Geometry check sheet. Reference: drawing and pictorial views, mm from the part's lowest x, y, z. A direction names the side the tool comes from. Give positions to 0.01 mm unless a question says otherwise; leave off trailing zeros. Write each loop counter-clockwise with the first axis right and the second up, starting at its lowest first coordinate (ties: lowest second). Pieces come first, ordered by that corner, then holes. Notation, with made-up numbers: (-11.5, 86.5) -> (17.5, 86.5) arc R29 cw to (17.5, 106.5) -> close; hole circle Ø2 at (77.5, -5.75). An arc over 180 degrees is marked (long way). Return JSON: item names as keys, results as strings.
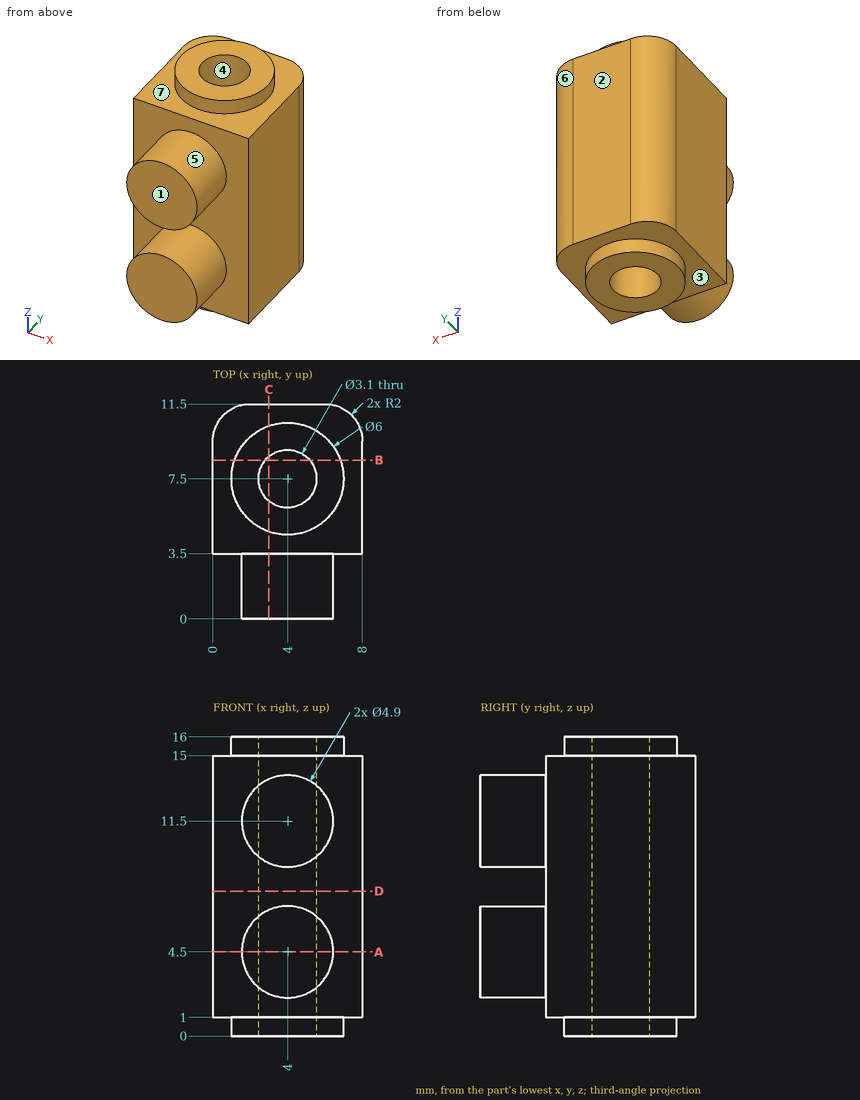
(1) Cross-section at D-D on z = 7.75. Enter the section's corners in (x, y).
Reply:
{"outline": "(0, 3.5) -> (8, 3.5) -> (8, 9.5) arc R2 ccw to (6, 11.5) -> (2, 11.5) arc R2 ccw to (0, 9.5) -> close; hole circle Ø3.1 at (4, 7.5)"}
(2) Cross-section at B-B on y = 8.5. Enter the section's corners in (x, z), then the cut area to 3 significant figures.
Reply:
{"outline": "(0, 1) -> (1.17, 1) -> (1.17, 0) -> (2.82, 0) -> (2.82, 16) -> (1.17, 16) -> (1.17, 15) -> (0, 15) -> close; (5.18, 0) -> (6.83, 0) -> (6.83, 1) -> (8, 1) -> (8, 15) -> (6.83, 15) -> (6.83, 16) -> (5.18, 16) -> close", "area": "85.4 mm^2"}
(3) Thickness scan on L1, parallel to Y at x = 4, z = 12; L2, parallel to Y at x = 2.75, z = 9; L3, parallel to X at y = 6.75, z = 13. Record the ranges inside material, lowest first.
Reply:
{"L1": "0 to 5.95, 9.05 to 11.5", "L2": "3.5 to 6.58, 8.42 to 11.5", "L3": "0 to 2.64, 5.36 to 8"}
(4) Set-up check for the marked faces 5, 6 and 7: record each of +Z, -Z, +X, -X, +Y, -Y from which the full face is reachable in a straight line by a thin tool's end or side.
Reply:
{"face 5": "-Y", "face 6": "+Z, -Z, +X, +Y", "face 7": "+Z"}
(5) Release check for a two-part mould opening along Y. For the marked faces 1, 2, 3 and 4 record: pulls with the +Y half, pulls with the -Y half, needs draft (parallel to the pull), parting line crosses it, or undercut.
Reply:
{"face 1": "pulls with the -Y half", "face 2": "pulls with the +Y half", "face 3": "needs draft", "face 4": "undercut"}
(6) Cross-section at A-A on z = 4.5. Enter the section's corners in (x, y).
Reply:
{"outline": "(0, 3.5) -> (1.55, 3.5) -> (1.55, 0) -> (6.45, 0) -> (6.45, 3.5) -> (8, 3.5) -> (8, 9.5) arc R2 ccw to (6, 11.5) -> (2, 11.5) arc R2 ccw to (0, 9.5) -> close; hole circle Ø3.1 at (4, 7.5)"}
(7) Cross-section at C-C on x = 3. Enter the section's corners in (y, z).
Reply:
{"outline": "(0, 2.26) -> (3.5, 2.26) -> (3.5, 1) -> (4.67, 1) -> (4.67, 0) -> (6.32, 0) -> (6.32, 16) -> (4.67, 16) -> (4.67, 15) -> (3.5, 15) -> (3.5, 13.74) -> (0, 13.74) -> (0, 9.26) -> (3.5, 9.26) -> (3.5, 6.74) -> (0, 6.74) -> close; (8.68, 0) -> (10.33, 0) -> (10.33, 1) -> (11.5, 1) -> (11.5, 15) -> (10.33, 15) -> (10.33, 16) -> (8.68, 16) -> close"}
